The drawing under review shows one solid part. Ordinate dimensions are in mm from its lowest x, y, z. A direction names the side the tool comes from. Coordinates: 2 decimals unless noted, no trailing zeros. Loops run counter-clockwise (first coordinate to the right, second up) from the corner with the lowest first, then second, coordinate; pieces in that order, holes last. Notation, with made-up numbers: M -22.5,85.25 L -13.5,85.25 A35 cw -13.5,121.25 Z; hole C -29.5,-31.75 d7. An arc over 180 degrees is marked long. Return JSON: item names as keys, results as strings.
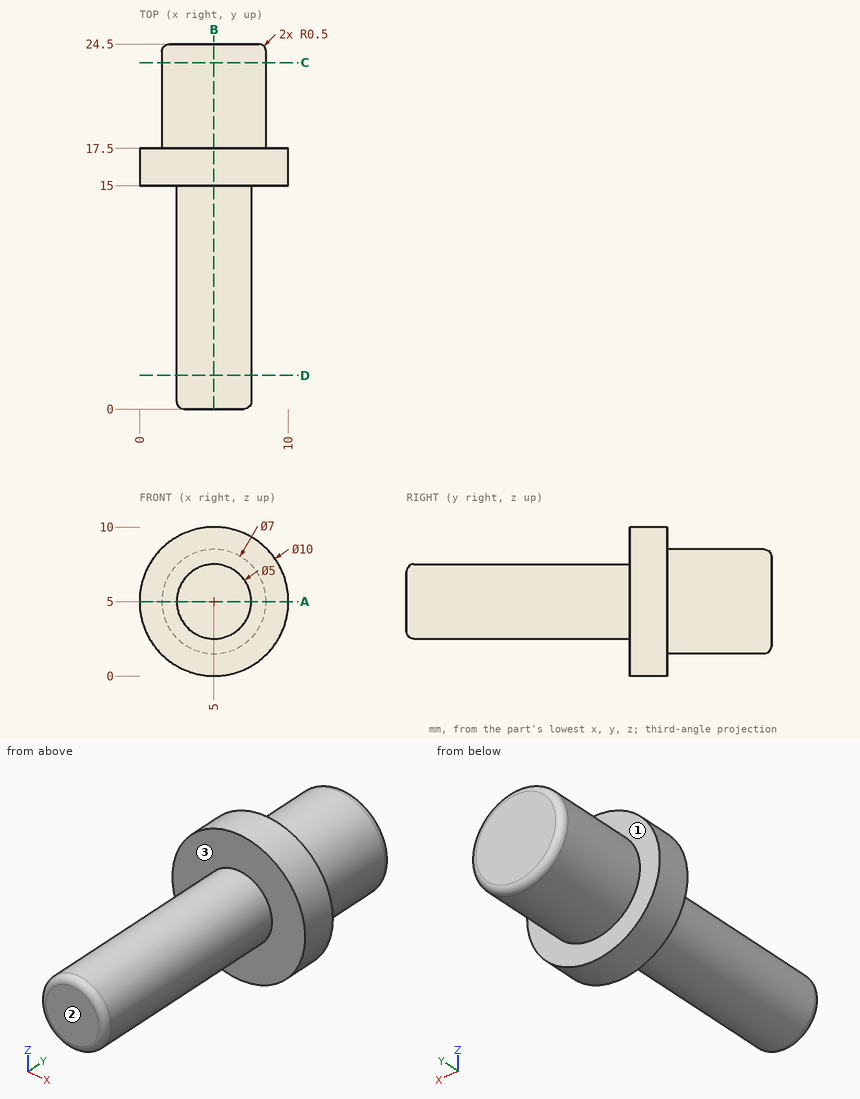
1. Insertion check: pin 1 Ø2 at (y, z) = (3.5, 3.5) entering from -X; pin 2 Ø3 at (y, z) = (11.5, 6) entering from -X; pin 3 Ø1.5 at (y, z) = (22, 4.5) entering from -X. Each pin has a flat end and moves straight along its axis. Give the tip position at first contact, or say it passes through.
Check values:
{"pin 1": "x = 2.55", "pin 2": "x = 2.5", "pin 3": "x = 1.5"}
2. Machinability: for the marked faces 1, 2 and 3, which of the approach directions +Z, -Z, +X, -X, +Y, -Y give a long, thin tool a straight path to every point of the face, cutting with its end or side? Answer none if there is none.
Check values:
{"face 1": "+Y", "face 2": "+Z, -Z, +X, -X, -Y", "face 3": "-Y"}
3. Add section A-A on z = 5. Give the boundary of the cut face in (x, y), plus the area to 3 significant figures.
Check values:
{"outline": "M 0,15 L 2.5,15 L 2.5,0.5 A0.5 ccw 3,0 L 7,0 A0.5 ccw 7.5,0.5 L 7.5,15 L 10,15 L 10,17.5 L 8.5,17.5 L 8.5,24 A0.5 ccw 8,24.5 L 2,24.5 A0.5 ccw 1.5,24 L 1.5,17.5 L 0,17.5 Z", "area": "149 mm²"}
4. Add section D-D on y = 2.25. Give the boundary of the cut face in (x, z), plus the area to 3 significant figures.
Check values:
{"outline": "C 5,5 d5", "area": "19.6 mm²"}
5. Add section B-B on x = 5. Give the boundary of the cut face in (y, z).
Check values:
{"outline": "M 0,3 A0.5 ccw 0.5,2.5 L 15,2.5 L 15,0 L 17.5,0 L 17.5,1.5 L 24,1.5 A0.5 ccw 24.5,2 L 24.5,8 A0.5 ccw 24,8.5 L 17.5,8.5 L 17.5,10 L 15,10 L 15,7.5 L 0.5,7.5 A0.5 ccw 0,7 Z"}
6. Add section C-C on y = 23.25. Give the boundary of the cut face in (x, z), plus the area to 3 significant figures.
Check values:
{"outline": "C 5,5 d7", "area": "38.5 mm²"}
7. To check wall thickness, follow line 1 (Y direction, x = 8.75, z = 1.75); line 2 (Y direction, x = 7, z = 6.75); line 3 (X direction, y = 5.25, z = 6.5). State the ranges of each line that lie inside material, in increasing order.
Check values:
{"line 1": "15 to 17.5", "line 2": "15 to 24.5", "line 3": "3 to 7"}
